Read the model definition and answer for the solid it produces. Units are mm, in the model's axes. Round coordinates to 2 decimals unless told otherwise and drop trailing zeros. Order: outer loops, then holes, each group sorted by start corner. A loop starts at its lowest first (then second) coordinate and runs counter-clockwise, first axis right, second up. Notation, with made-up numbers: (27, 66.25) -> (45, 66.25) arc R28 ccw to (45, 99.25) -> close; hole circle Ø4 at (33, -35). An arc over 180 degrees is marked (long way). Use a Markdown table: item, result. Add a question column.
1. Given pin 1 (2.5 mm diameter, centred on x = 199, z = 2, fed in from +Y); pin 2 (1.5 mm diameter, centred on y = -197.5, z = 3.5, fed in from -X); pin 3 (2.5 mm diameter, centred on x = -235.5, z = 2, fed in from +Y), each flat-ended and moving along its own axis, determine where each tip first touches the part or whether it passes through.
2. Consider L1, parallel to Y at x = -195, z = 1.6. Determine where the line is inside the solid, lowest interval first. Write a range as [from, to].
3. Section A-A, the plane z = 4.05 is taken. Give the vertices of the cut face in (x, y), then the cut area to 3 significant figures.
4. Section B-B, the plane y = -184 is taken. Give the vertices of the cut face in (x, z).
```python
from build123d import *

# Parameters (mm, degrees)
SALIENTE_EXTRUIR1_DEPTH = 5


with BuildPart() as part:
    # Croquis1 → Saliente-Extruir1 (new body)
    with BuildSketch(Plane.XY):
        Polygon((0, 246), (0, 0), (246, 0), (246, 176), (216, 176), (216, 216), (176, 216), (176, 246), align=None)
        Polygon((-246, 176), (-246, 0), (0, 0), (0, 246), (-176, 246), (-176, 216), (-216, 216), (-216, 176), align=None)
        Polygon((0, 0), (-246, 0), (-246, -176), (-216, -176), (-216, -216), (-176, -216), (-176, -246), (176, -246), (176, -216), (216, -216), (216, -176), (246, -176), (246, 0), align=None)
    extrude(amount=SALIENTE_EXTRUIR1_DEPTH)


solid = part.part
```
Verdict:
| question | item | result |
|---|---|---|
| 1 | pin 1 | stops at y = 216 |
| 1 | pin 2 | stops at x = -216 |
| 1 | pin 3 | stops at y = 176 |
| 2 | L1 | y = [-216, 216] |
| 3 | outline | (-246, -176) -> (-216, -176) -> (-216, -216) -> (-176, -216) -> (-176, -246) -> (176, -246) -> (176, -216) -> (216, -216) -> (216, -176) -> (246, -176) -> (246, 176) -> (216, 176) -> (216, 216) -> (176, 216) -> (176, 246) -> (-176, 246) -> (-176, 216) -> (-216, 216) -> (-216, 176) -> (-246, 176) -> close |
| 3 | area | 229,000 mm2 |
| 4 | outline | (-216, 0) -> (216, 0) -> (216, 5) -> (-216, 5) -> close |
